from build123d import *

# Parameters (mm, degrees)
F1_DEPTH = 4
F2_DEPTH = 80


with BuildPart() as f1:
    # F0 (on Top) → F1 (new body)
    with BuildSketch(Plane.XY):
        Polygon((-30.405549, -3.134592), (-12.488138, -27.899274), (17.343104, -24.823888), (30.364717, 3.130383), (11.913831, 27.840067), (-17.917411, 24.764681), align=None)
    extrude(amount=F1_DEPTH)

    # F0 (on Top) → F2 (join)
    with BuildSketch(Plane.XY):
        Polygon((13.76108, 32.051705), (-20.624834, 28.506766), (-35, -3.608247), (-14.375166, -32.115013), (20.010747, -28.570073), (35, 3.608247), align=None)
        Polygon((17.343104, -24.823888), (-12.488138, -27.899274), (-30.405549, -3.134592), (-17.917411, 24.764681), (11.913831, 27.840067), (30.364717, 3.130383), align=None, mode=Mode.SUBTRACT)
    extrude(amount=F2_DEPTH)


solid = f1.part
The listing builds one solid part. Answer for the finished solid, in the listing's coordinates (mm). A direction names the side the tool comes from. Coordinates: 2 decimals unless noted, no trailing zeros. Write each loop counter-clockwise with the first axis right and the second up, starting at its lowest first coordinate (ties: lowest second). Pieces come first, ordered by that corner, then holes. Notation, with made-up numbers: (48.25, -15) - (92.25, -15) arc R10 ccw to (92.25, 4) - close; hole circle Ø3 at (-16.75, 35.25). An arc over 180 degrees is marked (long way). Return JSON: item names as keys, results as strings.
1. For a pull along Y with two mould halves and no side action, classify faces 1 (the face through (2.64, -26.34, 41.47)), 2 (the face through (-3.191, 30.304, 39.44)), 3 (the face through (-21, -17, 80)) as +Y half, -Y half, draft (parallel to the pull), parting line (faces both ways), or undercut.
Final values:
{"face 1": "undercut", "face 2": "+Y half", "face 3": "draft"}
2. Each of these flat-tipped pins is pushed along its axis until it touches: pin 1 Ø3 at (x, z) = (21, 10) entering from +Y; pin 2 Ø1 at (y, z) = (-21, 24) entering from -X; pin 3 Ø12 at (x, z) = (25.5, 33.5) entering from -Y; pin 4 Ø12 at (x, z) = (-19.5, 38.5) entering from -Y (3 decimals). Where does it stop, or does it pass through?
Final values:
{"pin 1": "y = 24.37", "pin 2": "x = -22.78", "pin 3": "y = -28.62", "pin 4": "y = -32.115"}
3. Which of the six approach directions +Z, -Z, +X, -X, +Y, -Y give full straight-line access (tool end or side, diameter ignored) to faces 4 (the face through (-27.7, 12.7, 39.4)), 5 (the face through (23.945, -10.651, 41.468))?
Final values:
{"face 4": "+Z, -Z, -X, +Y", "face 5": "+Z"}
4. The part is cut by section C-C on x = 26.5. Determine the outline of the cut face in (y, z).
Final values:
{"outline": "(-14.64, 0) - (14.99, 0) - (14.99, 80) - (8.31, 80) - (8.31, 4) - (-5.17, 4) - (-5.17, 80) - (-14.64, 80) - close"}
5. The part is cut by section B-B on y = -11. Determine the outline of the cut face in (x, z), then the cut area to 3 significant figures.
Final values:
{"outline": "(-29.65, 0) - (28.2, 0) - (28.2, 80) - (23.78, 80) - (23.78, 4) - (-24.71, 4) - (-24.71, 80) - (-29.65, 80) - close", "area": "942 mm^2"}
6. The part is cut by section A-A on z = 17.5. Determine the outline of the cut face in (x, y).
Final values:
{"outline": "(-35, -3.61) - (-14.38, -32.12) - (20.01, -28.57) - (35, 3.61) - (13.76, 32.05) - (-20.62, 28.51) - close; hole (-30.41, -3.13) - (-12.49, -27.9) - (17.34, -24.82) - (30.36, 3.13) - (11.91, 27.84) - (-17.92, 24.76) - close"}
7. Consider line 1 along Z through (x, y) = (-5, -23); line 2 along X through (y, z) = (-4.5, 55); line 3 along Y through (x, z) = (10, 19). Determine where each line is inside the solid, lowest interval first.
Final values:
{"line 1": "0 to 4", "line 2": "-34.35 to -29.42, 26.81 to 31.22", "line 3": "-29.6 to -25.58, 27.64 to 31.66"}
